Study the drawing (mm; zero at the part's minimum x, y, z) and answer. A direction names the side the tool comes from. Give positions to 0.01 mm unless a question says otherwise; leave off trailing zeros. Write each loop counter-clockwise with the first axis right and the second up, starting at its lowest first coordinate (ties: lowest second). Pieces come first, ordered by that corner, then holes. Notation, with made-up numbers: M -18,-9 L 38,-9 A21 cw 38,27 Z; hole C 17,82.5 d5. An arc over 180 degrees is marked long. Use a Markdown table: item, result. Add a question column.
Item 1: Given P1, Ø4, axis at x = 26.5, z = 8.5, coming from the +Y side; P2, Ø1.5, axis at x = 7, z = 7, coming from the -Y side; P3, Ø6, axis at x = 11.5, z = 18.5, coming from the -Y side, each flat-ended and moving along its own axis, determine where each tip first touches the part or whether it passes through.
Item 2: The mould has two halves that part along X. Classify the marked faces 3, 4 and 5: pulls with the +X half, pulls with the -X half, needs draft (parallel to the pull), parting line crosses it, or undercut.
Item 3: A cutting plane is placed at A-A on x = 16. Determine the outline of the cut face in (y, z), then the cut area to 3 significant figures.
Item 4: A cutting plane is placed at C-C on z = 9.25. Determine the outline of the cut face in (x, y).
Item 5: For the marked faces 1 and 2, determine the directions among +Z, -Z, +X, -X, +Y, -Y from which every point of the face is accessible in a straight line to the end or side of a thin tool.
Item 6: Consider probe 1 along Y at (x, z) = (16, 11.25); probe 2 along Y at (x, z) = (12, 8); probe 3 along Z at (x, y) = (27.5, 14). Determine where each line is inside the solid, lowest interval first. Write a range as [from, to].
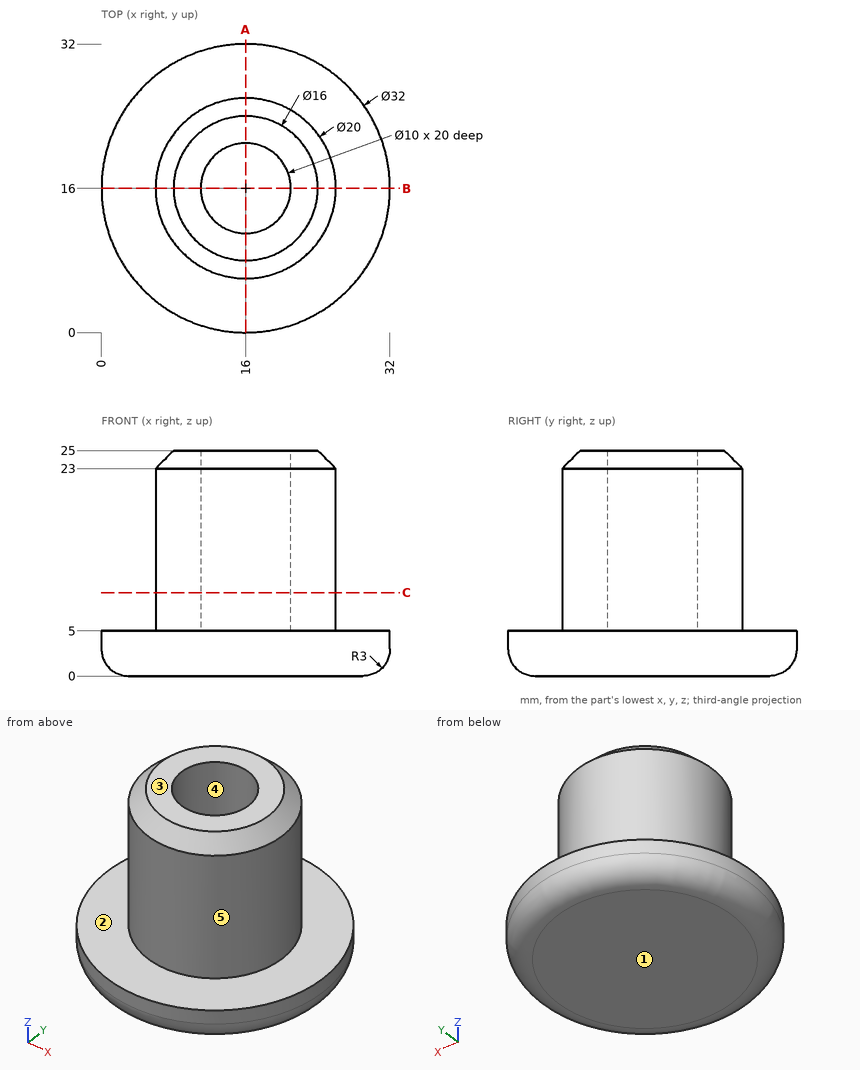
Filled in:
| question | item | result |
|---|---|---|
| 1 | P1 | y = 21.27 |
| 1 | P2 | y = 10.35 |
| 1 | P3 | y = 6.11 |
| 2 | face 3 | needs draft |
| 2 | face 4 | undercut |
| 2 | face 5 | parting line crosses it |
| 3 | outline | M 0,3 A3 ccw 3,0 L 29,0 A3 ccw 32,3 L 32,5 L 26,5 L 26,23 L 24,25 L 21,25 L 21,5 L 11,5 L 11,25 L 8,25 L 6,23 L 6,5 L 0,5 Z |
| 3 | area | 352 mm² |
| 4 | outline | C 16,16 d20; hole C 16,16 d10 |
| 5 | face 1 | -Z, +X, -X, +Y, -Y |
| 5 | face 2 | +Z |
| 6 | probe 1 | [6, 11], [21, 26] |
| 6 | probe 2 | [6.83, 13], [19, 25.17] |
| 6 | probe 3 | [0, 5] |
